Design review of the part built by this model. Coordinates are the model's own, in mm. A direction names the side the tool comes from. Coordinates: 2 decimals unless noted, no trailing zeros. Write each loop counter-clockwise with the first axis right and the second up, starting at its lowest first coordinate (ties: lowest second). Pieces come first, ordered by that corner, then holes.
Q1. For faces 5 (the flat face through (45.25, -2, 59)), 6 (the flat face through (-39, -28, 28)), list the 3-axis set-ups (+Z, -Z, +X, -X, +Y, -Y) from which the entire face can be reached by the end or side of a thin tool; tool diameter is ignored.
Q2. Take a section at A-A, the plane z = 39. Write out the cut boundary in (x, y), plus the area to 3 significant figures.
Q3. Take a section at C-C, the plane x = 17.5. Write out the cut boundary in (y, z), plus the area to 3 significant figures.
Q4. Take a section at B-B, the plane y = -20. Write out the cut boundary in (x, z), plus the area to 3 significant figures.
Q5. The part is to be moulded in two halves that separate along Y. For faces 1 (the flat face through (-41, 70, 28)), 2 (the flat face through (-39, 68, 28)), 3 (the flat face through (-41, -30, 28)), 4 (the flat face through (-124.75, -2, 59)), say which applies: released by +Y, released by -Y, zero draft, split by the parting line, or undercut.
Q6. For pin 1 Ø2 at (x, y) = (-32, -29.5) entering from +Z; pin 2 Ø1.6 at (x, y) = (-3.5, -29) entering from +Z; pin 3 Ø1 at (x, z) = (-80.5, 58.5) entering from -Y, all flat-tipped, find the tip position at first contact; note any pin that passes through.
Q7. For L1, parallel to Y at x = -34, z = 48; L2, parallel to Y at x = -18, z = 8.5, list the stretches that pass through material, from the lowest coordinate up.
from build123d import *

# Parameters (mm, degrees)
PAD001_DEPTH    = 250
SKETCH_W        = 170
SKETCH_H        = 100
PAD_DEPTH       = 60
FILLET_R        = 3
SKETCH001_W     = 17
SKETCH001_H     = 14.3
SKETCH001_W_2   = 15.6
SKETCH001_H_2   = 16.5
POCKET_DEPTH    = 45.251
SKETCH002_W     = 8.2
SKETCH002_H     = 4.6
POCKET001_DEPTH = 30.001
SKETCH006_W     = 165
SKETCH006_H     = 92
POCKET003_DEPTH = 500
SKETCH007_R     = 2.2
SKETCH007_R_2   = 1.75
POCKET004_DEPTH = 5


with BuildPart() as top_mask:
    # Sketch003 → Pad001 (new body, symmetric)
    with BuildSketch(Plane.YZ):
        with BuildLine():
            Line((-28, 0), (-28, 56.999991))
            ThreePointArc((-27, 58), (-27.70711, 57.707103), (-28, 56.999991))
            Line((-27, 58), (67, 58))
            ThreePointArc((68, 56.999991), (67.70711, 57.707103), (67, 58))
            Line((68, 0), (68, 56.999991))
            Line((-28, 0), (68, 0))
        make_face()
    extrude(amount=PAD001_DEPTH, both=True)


with BuildPart() as top:
    # Sketch → Pad (new body)
    with BuildSketch(Plane.XY):
        with Locations((-39.75, 20)):
            Rectangle(SKETCH_W, SKETCH_H)
    extrude(amount=PAD_DEPTH)

    # Fillet
    fillet_edges = [top.edges().sort_by_distance(p)[0] for p in [
        (45.25, 20, 0),
        (-39.75, -30, 60),
        (-39.75, 70, 60),
        (-124.75, 20, 0),
    ]]
    fillet(fillet_edges, radius=FILLET_R)

    # Sketch001 → Pocket (cut, through all)
    with BuildSketch(Plane.YZ):
        with Locations((-17.8, 14.75)):
            Rectangle(SKETCH001_W, SKETCH001_H)
        with Locations((1.05, 16.2)):
            Rectangle(SKETCH001_W_2, SKETCH001_H_2)
        with Locations((19, 16.2)):
            Rectangle(SKETCH001_W_2, SKETCH001_H_2)
    extrude(amount=POCKET_DEPTH, mode=Mode.SUBTRACT)

    # Sketch002 → Pocket001 (cut, through all)
    with BuildSketch(Plane.XZ):
        with BuildLine():
            ThreePointArc((-34.67, 11.2), (-35.73066, 10.76066), (-36.17, 9.7))
            Line((-36.17, 8.74), (-36.17, 9.7))
            ThreePointArc((-36.17, 8.74), (-35.73066, 7.67934), (-34.67, 7.24))
            Line((-27.93, 7.24), (-34.67, 7.24))
            ThreePointArc((-27.93, 7.24), (-26.86934, 7.67934), (-26.43, 8.74))
            Line((-26.43, 9.7), (-26.43, 8.74))
            ThreePointArc((-26.43, 9.7), (-26.86934, 10.76066), (-27.93, 11.2))
            Line((-34.67, 11.2), (-27.93, 11.2))
        make_face()
        with Locations((-16.704733, 9.1)):
            Rectangle(SKETCH002_W, SKETCH002_H)
        with Locations((-3.304733, 9.1)):
            Rectangle(SKETCH002_W, SKETCH002_H)
    extrude(amount=POCKET001_DEPTH, mode=Mode.SUBTRACT)

    # Sketch006 → Pocket003 (cut)
    with BuildSketch(Plane.XY.offset(30)):
        with Locations((-39.75, 20)):
            Rectangle(SKETCH006_W, SKETCH006_H)
    extrude(amount=POCKET003_DEPTH, mode=Mode.SUBTRACT)

    # Sketch007 → Pocket004 (cut)
    with BuildSketch(Plane.XY):
        with Locations((-39, 24.5)):
            Circle(SKETCH007_R)
        with Locations((19, 24.5)):
            Circle(SKETCH007_R)
        with Locations((-39, -24.5)):
            Circle(SKETCH007_R)
        with Locations((19, -24.5)):
            Circle(SKETCH007_R)
        with Locations((-112, 18.5)):
            Circle(SKETCH007_R)
        with Locations((-116.75, -23.9)):
            Circle(SKETCH007_R_2)
        with Locations((-116.75, 63.9)):
            Circle(SKETCH007_R_2)
        with Locations((37.25, 63.9)):
            Circle(SKETCH007_R_2)
    extrude(amount=POCKET004_DEPTH, mode=Mode.SUBTRACT)

    # Cut: cut Top Mask
    add(top_mask.part, mode=Mode.SUBTRACT)


solid = top.part
Responses:
1. face 5: +Z, -Z, +X, +Y, -Y
1. face 6: -Z, +X, -X
2. outline: (-124.75, -30) - (45.25, -30) - (45.25, -28) - (-124.75, -28) - close; (-124.75, 68) - (45.25, 68) - (45.25, 70) - (-124.75, 70) - close
2. area: 680 mm2
3. outline: (-30, 0) - (-28, 0) - (-28, 57) arc R1 cw to (-27, 58) - (-26, 58) - (-26, 60) - (-27, 60) arc R3 ccw to (-30, 57) - close; (66, 58) - (67, 58) arc R1 cw to (68, 57) - (68, 0) - (70, 0) - (70, 57) arc R3 ccw to (67, 60) - (66, 60) - close
3. area: 245 mm2
4. outline: (-124.75, 58) - (-122.25, 58) - (-122.25, 60) - (-124.75, 60) - close; (42.75, 58) - (45.25, 58) - (45.25, 60) - (42.75, 60) - close
4. area: 10.0 mm2
5. face 1: released by +Y
5. face 2: undercut
5. face 3: released by -Y
5. face 4: zero draft
6. pin 1: stops at z = 59.6
6. pin 2: stops at z = 59.75
6. pin 3: stops at y = -29.83
7. L1: y = -30 to -28, 68 to 70
7. L2: y = 68 to 70
